from build123d import *

# Parameters (mm, degrees)
F0_W     = 30.48
F0_H     = 7.62
F0_W_2   = 19.05
F0_H_2   = 3.556
F1_DEPTH = 10.16
F2_W     = 19.05
F2_H     = 3.556
F3_DEPTH = 6.096
F4_R     = 1.27


with BuildPart() as f1:
    # F0 (on Right) → F1 (new body)
    with BuildSketch(Plane.YZ):
        Rectangle(F0_W, F0_H)
        Rectangle(F0_W_2, F0_H_2, mode=Mode.SUBTRACT)
        Rectangle(F0_W_2, F0_H_2)
    extrude(amount=-F1_DEPTH)

    # F2 (on face) → F3 (join)
    with BuildSketch(Plane.YZ):
        Rectangle(F2_W, F2_H)
    extrude(amount=F3_DEPTH)

    # F4
    f4_edges = [f1.edges().sort_by_distance(p)[0] for p in [
        (6.096, 0, 1.778),
        (6.096, -9.525, 0),
        (6.096, 0, -1.778),
        (6.096, 9.525, 0),
    ]]
    fillet(f4_edges, radius=F4_R)


solid = f1.part
Model file for the job. Use its own axes, mm. A direction names the side the tool comes from. Round coordinates to 2 decimals unless told otherwise and drop trailing zeros. Loops run counter-clockwise (first coordinate to the right, second up) from the corner with the lowest first, then second, coordinate; pieces in that order, holes last. Notation, with made-up numbers: (61, -12.5) - (103, -12.5) arc R29 ccw to (103, 24.5) - close; hole circle Ø9 at (76, 74.5). An arc over 180 degrees is marked (long way). Write each question's results on one line, items separated by ' | '.
(1) Saw through at A-A, the plane y = 1.5. List the corners of the cut face in (x, z).
Answer below:
outline: (-10.16, -3.81) - (0, -3.81) - (0, -1.78) - (4.83, -1.78) arc R1.27 ccw to (6.1, -0.51) - (6.1, 0.51) arc R1.27 ccw to (4.83, 1.78) - (0, 1.78) - (0, 3.81) - (-10.16, 3.81) - close
(2) Pin check, flat tips, straight feed: pin 1 (2.5 mm diameter, centred on x = 2.5, y = -2, fed in from +Z); pin 2 (1.1 mm diameter, centred on x = 2.5, z = 1, fed in from +Y) (3 decimals); pin 3 (5.5 mm diameter, centred on x = 1.5, y = 1.5, fed in from -Z); pin 4 (4 mm diameter, centred on x = 3, z = 0.5, fed in from -Y) (3 decimals). Stop position of each tip, or through.
Answer below:
pin 1: stops at z = 1.78 | pin 2: stops at y = 9.525 | pin 3: stops at z = -3.81 | pin 4: stops at y = -9.525
(3) Wall check: L1, parallel to X at y = -7.5, z = -3; L2, parallel to Z at x = 3.25, y = 2; L3, parallel to Y at x = 1.5, z = -1.25 (3 decimals). Give the ranges that are in metal, low to high.
Answer below:
L1: x = -10.16 to 0 | L2: z = -1.78 to 1.78 | L3: y = -9.525 to 9.525
(4) Saw through at C-C, the plane y = 12.5. List the corners of the cut face in (x, z), then the cut area to 3 significant figures.
Answer below:
outline: (-10.16, -3.81) - (0, -3.81) - (0, 3.81) - (-10.16, 3.81) - close | area: 77.4 mm^2
(5) 3-axis set-ups, long thin cutter, end or side, ignore diameter. For faces 1 (the flat face through (2, 0, -1.778)), 2 (the flat face through (-10.16, 0, 0)), 3 (the flat face through (2, -9.525, 0)), 4 (the flat face through (2, 0, 1.778)), 5 (the flat face through (2, 9.525, 0)): which of +Z, -Z, +X, -X, +Y, -Y reach the whole face in a straight line?
Answer below:
face 1: -Z, +X, +Y, -Y | face 2: +Z, -Z, -X, +Y, -Y | face 3: +Z, -Z, +X, -Y | face 4: +Z, +X, +Y, -Y | face 5: +Z, -Z, +X, +Y
(6) Saw through at B-B, the plane z = 0. List the corners of the cut face in (x, y) (3 decimals).
Answer below:
outline: (-10.16, -15.24) - (0, -15.24) - (0, -9.525) - (4.826, -9.525) arc R1.27 ccw to (6.096, -8.255) - (6.096, 8.255) arc R1.27 ccw to (4.826, 9.525) - (0, 9.525) - (0, 15.24) - (-10.16, 15.24) - close
